Read the model definition and answer for the solid it produces. Units are mm, in the model's axes. A direction names the side the tool comes from. Round coordinates to 2 decimals unless told otherwise and drop trailing zeros. Write each loop counter-clockwise with the first axis right and the second up, starting at its lowest first coordinate (ties: lowest second). Pieces come first, ordered by that corner, then holes.
from build123d import *

# Parameters (mm, degrees)
SKETCH_1_W          = 30
SKETCH_1_H          = 31
SKETCH_1_R          = 10.5
EXTRUDE_1_DEPTH     = 30
FILLET_1_R          = 15
FILLET_2_R          = 15
SKETCH_2_W          = 30
SKETCH_2_H          = 7
EXTRUDE_2_DEPTH     = 7
SKETCH_3_W          = 30
SKETCH_3_H          = 7
EXTRUDE_3_DEPTH     = 7
SKETCH_4_R          = 2
CUT_EXTRUDE_1_DEPTH = 7


with BuildPart() as part:
    # Эскиз1 → Бобышка-Вытянуть1 (new body)
    with BuildSketch(Plane.XY):
        with Locations((0, 15.5)):
            Rectangle(SKETCH_1_W, SKETCH_1_H)
        with Locations((0, 15)):
            Circle(SKETCH_1_R, mode=Mode.SUBTRACT)
    extrude(amount=EXTRUDE_1_DEPTH)

    # Скругление1
    fillet_1_edges = [part.edges().sort_by_distance(p)[0] for p in [
        (15, 0, 15),
    ]]
    fillet(fillet_1_edges, radius=FILLET_1_R)

    # Скругление2
    fillet_2_edges = [part.edges().sort_by_distance(p)[0] for p in [
        (-15, 0, 15),
    ]]
    fillet(fillet_2_edges, radius=FILLET_2_R - 0.0001)  # a hair under: the kernel refuses the full size

    # Эскиз2 → Бобышка-Вытянуть2 (add)
    with BuildSketch(Plane(origin=(15, 0, 0), x_dir=(0, 0, -1), z_dir=(1, 0, 0))):
        with Locations((-15, 27.5)):
            Rectangle(SKETCH_2_W, SKETCH_2_H)
    extrude(amount=EXTRUDE_2_DEPTH)

    # Эскиз3 → Бобышка-Вытянуть3 (add)
    with BuildSketch(Plane.ZY.offset(15)):
        with Locations((15, 27.5)):
            Rectangle(SKETCH_3_W, SKETCH_3_H)
    extrude(amount=EXTRUDE_3_DEPTH)

    # Эскиз4 → Вырез-Вытянуть1 (cut)
    with BuildSketch(Plane(origin=(0, 31, 0), x_dir=(1, 0, 0), z_dir=(0, 1, 0))):
        with Locations(Location((18.5, -3.5, 0), (0, 0, 270))):
            Circle(SKETCH_4_R)
        with Locations(Location((18.5, -26.5, 0), (0, 0, 270))):
            Circle(SKETCH_4_R)
        with Locations(Location((-18.5, -26.5, 0), (0, 0, 270))):
            Circle(SKETCH_4_R)
        with Locations(Location((-18.5, -3.5, 0), (0, 0, 270))):
            Circle(SKETCH_4_R)
    extrude(amount=-CUT_EXTRUDE_1_DEPTH, mode=Mode.SUBTRACT)


solid = part.part
Q1. Section B-B (x = 18.5) is taken. Determine the outline of the cut face in (y, z), then the cut area to 3 significant figures.
Verdict:
outline: (24, 0) - (31, 0) - (31, 1.5) - (24, 1.5) - close; (24, 5.5) - (31, 5.5) - (31, 24.5) - (24, 24.5) - close; (24, 28.5) - (31, 28.5) - (31, 30) - (24, 30) - close
area: 154 mm2
Q2. Straight lines are drawn through the part: probe 1 along X at (y, z) = (26.25, 3.5); probe 2 along Z at (x, y) = (18, 29); probe 3 along Y at (x, z) = (16.5, 23.25). For each, find the intervals that lie inside material, in ascending order.
Verdict:
probe 1: x = -22 to -20.5, -16.5 to 16.5, 20.5 to 22
probe 2: z = 0 to 1.56, 5.44 to 24.56, 28.44 to 30
probe 3: y = 24 to 31
Q3. Which of the six approach directions +Z, -Z, +X, -X, +Y, -Y give full straight-line access (tool end or side, diameter ignored) to faces 1 (the flat face through (18, 24, 15)), 2 (the flat face through (-15, 19, 15)), 3 (the flat face through (0, 31, 15))?
Verdict:
face 1: +Z, -Z, +X, -Y
face 2: +Z, -Z, -X, -Y
face 3: +Z, -Z, +X, -X, +Y
Q4. Flat-ended cylindrical pins translate along their axes: pin 1 Ø6.5 at (x, z) = (-18.5, 26.5) entering from -Y; pin 2 Ø5 at (x, z) = (18.5, 26.5) entering from +Y; pin 3 Ø4.5 at (y, z) = (21.5, 9.5) entering from -X; pin 4 Ø8 at (x, z) = (13, 12.5) entering from -Y. Find the tip coordinate at first contact, or state that the pin passes through.
Verdict:
pin 1: stops at y = 24
pin 2: stops at y = 31
pin 3: stops at x = -15
pin 4: stops at y = 3
Q5. Determine the mould class of faces 4 (the flat face through (15, 19, 15)), 5 (the cylindrical face through (10.49, 4.28, 15.21)), 6 (the cylindrical face through (-1.37, 25.41, 14.79)) for opening direction Y: pulls with the +Y half, pulls with the -Y half, needs draft (parallel to the pull), parting line crosses it, or undercut.
Verdict:
face 4: needs draft
face 5: pulls with the -Y half
face 6: undercut
Q6. Section D-D (x = -5) is taken. Determine the outline of the cut face in (y, z).
Verdict:
outline: (0.86, 0) - (5.77, 0) - (5.77, 30) - (0.86, 30) - close; (24.23, 0) - (31, 0) - (31, 30) - (24.23, 30) - close
Q7. Section A-A (z = 26.5) is taken. State how many separate pieces and enclosed holes the cut face has, then the cut area to 3 significant figures.
Verdict:
separate pieces: 3
enclosed holes: 1
area: 529 mm2
